from build123d import *

# Parameters (mm, degrees)
F1_DEPTH  = 8
F3_DEPTH  = 3
F3_TAPER  = 10
F4_SIZE   = 1
F5_W      = 2.5
F5_H      = 2.5
F6_DEPTH  = 2
F7_R      = 2.5
F8_DEPTH  = 5
F8_TAPER  = -30
F9_W      = 28.2842712475
F9_H      = 3.5
F10_DEPTH = 3.5
F11_W     = 28.2842712475
F11_H     = 3.5
F12_DEPTH = 3.5


with BuildPart() as f1:
    # F0 (on Top) → F1 (new body)
    with BuildSketch(Plane.XY):
        Polygon((0, 20), (0, 0), (20, 0), (40, 20), (40, 40), (20, 40), align=None)
    extrude(amount=F1_DEPTH)

    # F2 (on face) → F3 (cut)
    with BuildSketch(Plane.XY.offset(8)):
        Polygon((2, 19.1715728753), (2, 2), (19.1715728753, 2), (38, 20.8284271247), (38, 38), (20.8284271247, 38), align=None)
    extrude(amount=-F3_DEPTH, taper=F3_TAPER, mode=Mode.SUBTRACT)

    # F4
    f4_edges = [f1.edges().sort_by_distance(p)[0] for p in [
        (0, 0, 4),
        (40, 40, 4),
    ]]
    chamfer(f4_edges, length=F4_SIZE)

    # F5 (on face) → F6 (cut)
    with BuildSketch(Plane.XY.offset(8)):
        with Locations((1.25, 1.25)):
            Rectangle(F5_W, F5_H)
        with Locations((38.75, 38.75)):
            Rectangle(F5_W, F5_H)
    extrude(amount=-F6_DEPTH, mode=Mode.SUBTRACT)

    # F7 (on face) → F8 (cut, through all)
    with BuildSketch(Plane.XY.offset(5)):
        with Locations((12.5289809421, 12.5289809421)):
            Circle(F7_R)
        with Locations((27.4710190579, 27.4710190579)):
            Circle(F7_R)
    extrude(amount=-F8_DEPTH, taper=F8_TAPER, mode=Mode.SUBTRACT)

    # F9 (on face) → F10 (join)
    with BuildSketch(Plane(origin=(10, -10, 0), x_dir=(0.7071067812, 0.7071067812, 0), z_dir=(0.7071067812, -0.7071067812, 0))):
        with Locations((28.2842712475, 1.75)):
            Rectangle(F9_W, F9_H)
    extrude(amount=F10_DEPTH)

    # F11 (on face) → F12 (join)
    with BuildSketch(Plane(origin=(-10, 10, 0), x_dir=(-0.7071067812, -0.7071067812, 0), z_dir=(-0.7071067812, 0.7071067812, 0))):
        with Locations((-28.2842712475, 1.75)):
            Rectangle(F11_W, F11_H)
    extrude(amount=F12_DEPTH)


solid = f1.part
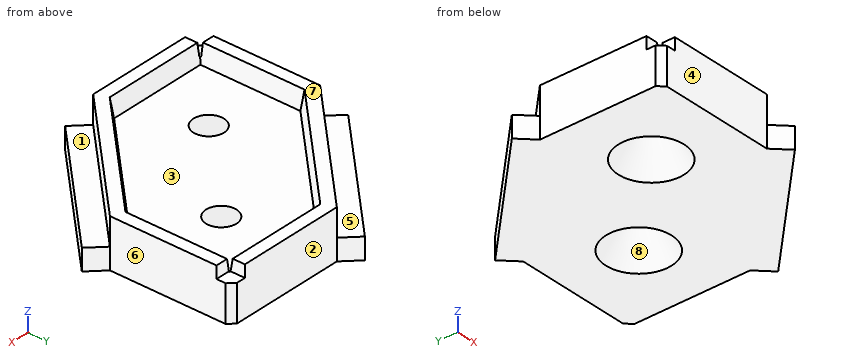
Check sheet for the modelled part. Datum: model origin and axes. Units: mm. Face numbers are marked on the shaded views. A direction names the side the tool comes from. Give positions to 0.01 mm unless a question says otherwise; leave off trailing zeros. Write each loop counter-clockwise with the first axis right and the second up, starting at its lowest first coordinate (ties: lowest second). Pieces come first, ordered by that corner, then holes. Notation, with made-up numbers: (-6, 4.25) -> (3, 4.25) arc R33 cw to (3, 43.25) -> close; hole circle Ø7 at (44.5, 79.5). An arc over 180 degrees is marked (long way). Use one line per item in the form item = value. Start each with the question number.
1. Mould release check, pull along X, two halves, no side actions. Record for the marked faces 6, 7 and 8: pulls with the +X half, pulls with the -X half, needs draft (parallel to the pull), parting line crosses it, or undercut.
2. Go/stop test with flat-tipped pins: P1, Ø4, axis at y = 26.5, z = 2, coming from the +X side; P2, Ø0.8, axis at x = 39, y = 39, coming from the +Z side; P3, Ø1, axis at y = 1.5, z = 7.5, coming from the -X side; P4, Ø24.5, axis at x = 34.5, y = 7, coming from the +Z side. Record where each tip stops, or that it passes through.
3. Thickness scan on line 1 along Z through (x, y) = (7.5, 4.5); line 2 along X through (y, z) = (5, 7.5); line 3 along X through (y, z) = (16.5, 6). Record the ranges inside material, lowest first. Write a range as from..to.
4. Access from +Z, -Z, +X, -X, +Y, -Y to the whole of each face (thin tool, end or side, straight path). Record for the marked faces 1, 2, 3, 4 and 5.
5. Section check A-A (z = 4.25). Record the cut outline in (x, y).
6. Section check B-B (z = 1.75). Record the cut outline in (x, y).
Conclusion:
q1.face_6 = pulls with the +X half
q1.face_7 = needs draft
q1.face_8 = undercut
q2.P1 = 40
q2.P2 = 6
q2.P3 = 2.5
q2.P4 = 8
q3.line_1 = 0..5
q3.line_2 = 0..2.09, 22.05..25
q3.line_3 = 0..2.35, 33.17..36.5
q4.face_1 = +Z, +X, -Y
q4.face_2 = +Z, -Z, +X, +Y
q4.face_3 = +Z
q4.face_4 = +Z, -Z, -X, -Y
q4.face_5 = +Z, -X, +Y
q5.outline = (0, 1) -> (1, 0) -> (20, 0) -> (40, 20) -> (40, 39) -> (39, 40) -> (20, 40) -> (0, 20) -> close; hole circle Ø5.87 at (12.53, 12.53); hole circle Ø5.87 at (27.47, 27.47)
q6.outline = (-2.47, 22.47) -> (0, 20) -> (0, 1) -> (1, 0) -> (20, 0) -> (22.47, -2.47) -> (42.47, 17.53) -> (40, 20) -> (40, 39) -> (39, 40) -> (20, 40) -> (17.53, 42.47) -> close; hole circle Ø8.75 at (12.53, 12.53); hole circle Ø8.75 at (27.47, 27.47)
